Answer from the drawing. Dimensions are ordinates in mm from the lowest x, y and z of the part. Round coordinates to 2 decimals unless told otherwise and drop trailing zeros. Order: outer loops, then holes, each group sorted by start corner. A loop starts at its lowest first (then second) coordinate and runs counter-clockwise, first axis right, second up. Notation, with made-up numbers: (-31.75, -39) -> (-22.75, -39) arc R27 cw to (-22.75, -1) -> close; hole circle Ø10 at (8.5, -14.5). An arc over 180 degrees is marked (long way). Use a Markdown table: item, result. Add a question column.
Item 1: A flat-ended cylindrical pin translates along its axis: P1, Ø1, axis at x = 61.5, y = 67, coming from the -Z side. Find the tip coordinate at first contact, or state that the pin passes through.
Item 2: A cutting plane is placed at A-A, the plane y = 56.5. Determine the outline of the cut face in (x, z), plus the area to 3 significant figures.
Item 3: Find the intervals of material crossed by L1, parallel to X at y = 57.5, z = 5; L2, parallel to Y at x = 204.97, z = 3.5; L3, parallel to Y at x = 13, z = 3, in increasing order. Write a range as [from, to].
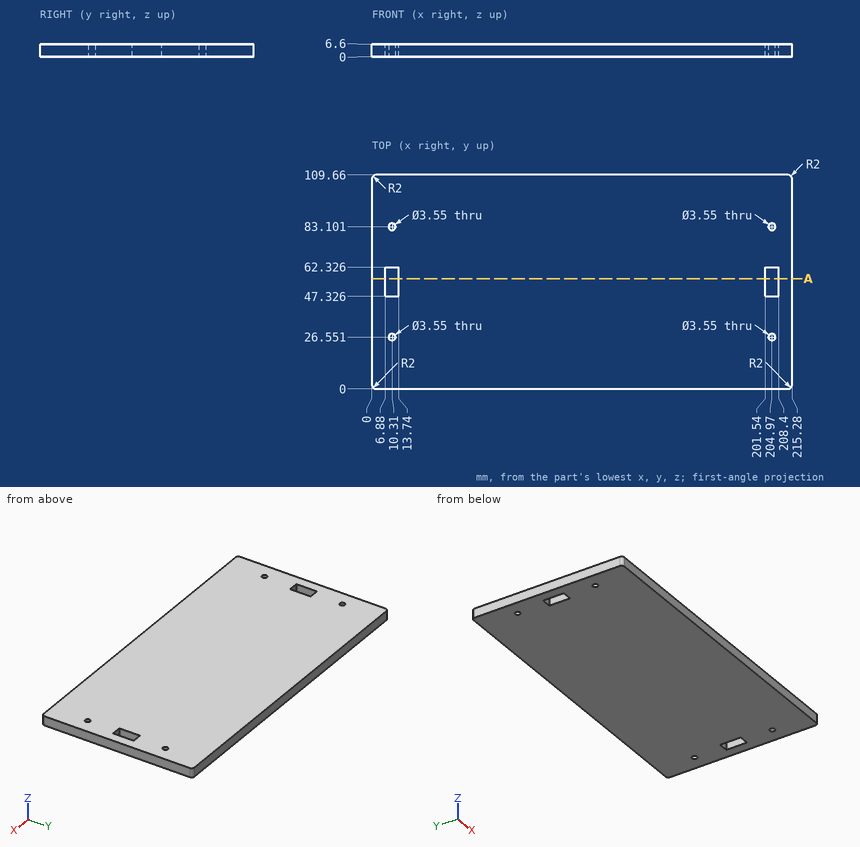
Reported:
| question | item | result |
|---|---|---|
| 1 | P1 | z = 0 |
| 2 | outline | (0, 0) -> (6.88, 0) -> (6.88, 6.6) -> (0, 6.6) -> close; (13.74, 0) -> (201.54, 0) -> (201.54, 6.6) -> (13.74, 6.6) -> close; (208.4, 0) -> (215.28, 0) -> (215.28, 6.6) -> (208.4, 6.6) -> close |
| 2 | area | 1,330 mm² |
| 3 | L1 | [0, 6.88], [13.74, 201.54], [208.4, 215.28] |
| 3 | L2 | [0, 24.78], [28.33, 47.33], [62.33, 81.33], [84.88, 109.66] |
| 3 | L3 | [0, 47.33], [62.33, 109.66] |
